Check sheet for the modelled part. Datum: model origin and axes. Units: mm. Face numbers are marked on the shaded views. A direction names the side the tool comes from. Round coordinates to 2 decimals unless told otherwise and drop trailing zeros. Order: outer loops, then holes, each group sorted by start corner. A loop starts at its lowest first (then second) coordinate and runs counter-clockwise, first axis right, second up.
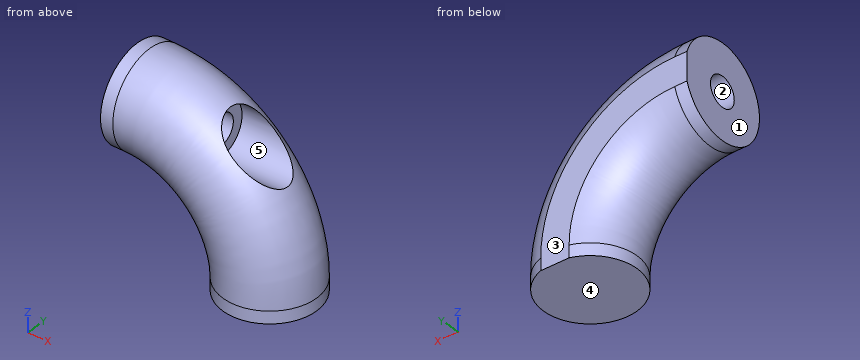
from build123d import *

# Parameters (mm, degrees)
F1_R      = 4.96
F3_R      = 1.5875
F4_DEPTH  = 18.961
F6_R      = 2.75
F7_DEPTH  = 10.16
F9_W      = 0.254
F9_H      = 19.05
F10_DEPTH = 18.961


with BuildPart() as f2:
    # F2: sweep along a path in F0
    with BuildLine(Plane.XZ) as f2_path:
        Line((0, 0), (1.3, 0))
        ThreePointArc((1.3, 0), (10.280256, -3.719744), (14, -12.7))
        Line((14, -12.7), (14, -14))
    # F1 (on Right) → F2 (sweep)
    with BuildSketch(Plane.YZ):
        Circle(F1_R)
    sweep(path=f2_path.line)

    # F3 (on face) → F4 (cut, through all)
    with BuildSketch(Plane(origin=(0, 0, 0), x_dir=(0, -1, 0), z_dir=(-1, 0, 0))):
        Circle(F3_R)
    extrude(amount=-F4_DEPTH, mode=Mode.SUBTRACT)

    # F6 (on offset) → F7 (cut)
    with BuildSketch(Plane.YZ.offset(19.05)):
        Circle(F6_R)
    extrude(amount=-F7_DEPTH, mode=Mode.SUBTRACT)

    # F9 (on Right) → F10 (cut, through all)
    with BuildSketch(Plane.YZ):
        with Locations((4.853686, -4.475)):
            Rectangle(F9_W, F9_H)
    extrude(amount=F10_DEPTH, mode=Mode.SUBTRACT)


solid = f2.part
1) Scan lines: line 1 (Z direction, x = 4, y = 0.5); line 2 (Y direction, x = 11.5, z = 0); line 3 (X direction, y = 0.5, z = -2.5). Record each from-to range of solid material in increasing order.
2) Set-up check for the marked faces 4 and 5: record each of +Z, -Z, +X, -X, +Y, -Y from which the full face is reachable in a straight line by a thin tool's end or side.
3) Gauge pin test, flat ends, axial feed: pin 1 (4 mm diameter, centred on x = 11, y = -2.5, fed in from +Z); pin 2 (4 mm diameter, centred on x = 6.5, z = -6, fed in from -Y). Record the tip position at first contact, or that the pin passes through.
4) Sectioned sample at A-A on y = 0. Record the cut outline in (x, z).
5) Sectioned sample at C-C on y = 1. Record the cut outline in (x, z), and give its area (3 significant figures).
6) Draft check along Y on the marked faces 1, 2 and 3. Enter one of: pulls with the +Y half, pulls with the -Y half, needs draft (parallel to the pull), parting line crosses it, or undercut.
7) Sectioned sample at B-B on y = -2. Record the cut outline in (x, z), and give its area (3 significant figures).
Values found:
1. line 1: z = -5.42 to -1.51, 1.51 to 4.73
1. line 2: y = -3.42 to -2.75, 2.75 to 3.42
1. line 3: x = 0 to 8.89
2. face 4: -Z, +X, -X, +Y, -Y
2. face 5: +X
3. pin 1: stops at z = 2.8
3. pin 2: stops at y = -4.44
4. outline: (0, -4.96) - (1.3, -4.96) arc R7.74 cw to (9.04, -12.7) - (9.04, -14) - (18.96, -14) - (18.96, -12.7) arc R17.66 ccw to (15.89, -2.75) - (8.89, -2.75) - (8.89, -1.59) - (0, -1.59) - close; (0, 1.59) - (8.89, 1.59) - (8.89, 2.75) - (9.85, 2.75) arc R17.66 ccw to (1.3, 4.96) - (0, 4.96) - close
5. outline: (0, -4.86) - (1.3, -4.86) arc R7.84 cw to (9.14, -12.7) - (9.14, -14) - (18.86, -14) - (18.86, -12.7) arc R17.56 ccw to (15.64, -2.56) - (8.89, -2.56) - (8.89, -1.23) - (0, -1.23) - close; (0, 1.23) - (8.89, 1.23) - (8.89, 2.56) - (9.98, 2.56) arc R17.56 ccw to (1.3, 4.86) - (0, 4.86) - close
5. area: 175 mm2
6. face 1: needs draft
6. face 2: undercut
6. face 3: pulls with the +Y half
7. outline: (0, -4.54) - (1.3, -4.54) arc R8.16 cw to (9.46, -12.7) - (9.46, -14) - (18.54, -14) - (18.54, -12.7) arc R17.24 ccw to (14.73, -1.89) - (8.89, -1.89) - (8.89, 1.89) - (10.49, 1.89) arc R17.24 ccw to (1.3, 4.54) - (0, 4.54) - close
7. area: 190 mm2
